Design review of the part built by this model. Coordinates are the model's own, in mm. A direction names the side the tool comes from. Give positions to 0.01 mm unless a question says otherwise; leave off trailing zeros. Write each loop counter-clockwise with the first axis right and the second up, starting at its lowest first coordinate (ties: lowest second). Pieces come first, ordered by that corner, then holes. Notation, with made-up numbers: (-23, 14.5) -> (8, 14.5) arc R30 cw to (8, 46.5) -> close; hole circle Ø2 at (87.5, -26). An arc over 180 degrees is marked (long way). Write each question's results on one line, items separated by ' | '. Start each with the question number.
(1) Mouldability with a two-part tool opening along Z and no side actions: class faces 1 (the face through (87, 1, 182)), 2 (the face through (80, 1, 195.7)), 3 (the face through (74, 0, 171)), 4 (the face through (80, 1, 197.7)) as released by +Z, released by -Z, zero draft, split by the parting line, or undercut.
(2) Take a section at A-A (z = 186). State the section outline as (x, y) points, plus the area to 3 significant figures.
(3) For faces 5 (the face through (71.4, 1, 190)), 6 (the face through (79.5, 2.2, 195.5)), list the 3-axis set-ups (+Z, -Z, +X, -X, +Y, -Y) from which the entire face can be reached by the end or side of a thin tool; tool diameter is ignored.
(4) Take a section at B-B (x = 81). State the section outline as (y, z) points.
(5) To check wall thickness, follow probe 1 along X at (y, z) = (0.35, 195); probe 2 along X at (y, z) = (0.3, 161); probe 3 along Z at (x, y) = (84, 0.9). State the ranges of each line that lie inside material, in increasing order.
(6) Take a section at D-D (z = 159). State the section outline as (x, y) points, plus the area to 3 significant figures.
(7) Take a section at C-C (y = 0.8). State the section outline as (x, z) points.
(8) Clearance check with flat-ended pins moving along their axes: pin 1 (1 mm diameter, centred on x = 83, z = 186, fed in from +Y); pin 2 (1.1 mm diameter, centred on x = 76.5, y = 1.5, fed in from -Z); pin 3 (1 mm diameter, centred on x = 85, y = 2, fed in from -Z); pin 4 (6 mm diameter, centred on x = 77, z = 185.5, fed in from -Y). State where each tip first meets the part, or that it passes through.
Autodesk Fusion 360 part; units mm, degrees
sketch "snippy-Edge_Cuts" plane through (0, 0, 0) normal (0, 1, 0) x (1, 0, 0)
  line L0 (73.4, -145) -> (85.6, -145)
  line L1 (85.6, -145) -> (85.6, -157)
  line L2 (85.6, -157) -> (73.4, -157)
  line L3 (73.4, -157) -> (73.4, -145)
  line L4 (73.4, -145) -> (73.4, -157)
  line L5 (73.4, -157) -> (85.6, -157)
  line L6 (85.6, -157) -> (85.6, -195.7)
  line L7 (85.6, -195.7) -> (73.4, -195.7)
  line L8 (73.4, -195.7) -> (73.4, -157)
  line L9 (87.6, -182) -> (87.6, -197.7)
  line L10 (87.6, -197.7) -> (71.4, -197.7)
  line L11 (71.4, -197.7) -> (71.4, -182)
  line L12 (73.4, -157) -> (85.6, -157)
  line L13 (84.5, -157) -> (74.5, -157)
  line L14 (74.5, -157) -> (74.5, -195.7)
  line L15 (74.5, -195.7) -> (84.5, -195.7)
  line L16 (84.5, -195.7) -> (84.5, -157)
  line L17 (85.6, -157) -> (85.6, -182)
  line L18 (85.6, -182) -> (87.6, -182)
  line L19 (87.6, -182) -> (71.4, -182)
  dimension "d4" = 12
  dimension "d8" = 12.2
  dimension "d9" = 12.2
  dimension "d23" = 10
  dimension "d25" = 1.1
  dimension "d26" = 1.1
extrude "Extrude6" add sketch "snippy-Edge_Cuts" along normal blind 0.4 contours L0 L1 L2 L3 L4 L5 L12 L13 | L2 L5 L8 L12 L14 L19 | L2 L5 L6 L12 L16 L17 L19 | L7 L8 L14 L19 | L6 L7 L8 L9 L10 L11 L15 L18 L19 | L6 L7 L16 L19 makes body 1
extrude "Extrude7" cut sketch "snippy-Edge_Cuts" along normal blind 2.6 contours L6 L7 L8 L9 L10 L11 L15 L18 L19 bodies 1
extrude "Extrude8" add sketch "snippy-Edge_Cuts" along normal blind 2.2 contours L6 L7 L8 L9 L10 L11 L15 L18 L19 bodies 1
extrude "Extrude9" add 1 faces at (77.4667, 2.2, 197.0333) along direction (0, 1, 0) blind 0.4 separate body on bodies 1 makes body 2
sketch "Sketch6" plane through (0, 2.6, 0) normal (0, 1, 0) x (-1, 0, 0)
  line L0 (-87.6, 197.7) -> (-87.6, 182)
  line L1 (-87.6, 182) -> (-85.6, 182)
  line L2 (-85.6, 182) -> (-85.6, 195.7)
  line L3 (-85.6, 195.7) -> (-73.4, 195.7)
  line L4 (-73.4, 195.7) -> (-73.4, 182)
  line L5 (-73.4, 182) -> (-71.4, 182)
  line L6 (-71.4, 182) -> (-71.4, 197.7)
  line L7 (-71.4, 197.7) -> (-87.6, 197.7)
  line L8 (-85.1, 182) -> (-85.1, 195.2)
  line L9 (-85.1, 195.2) -> (-73.9, 195.2)
  line L10 (-73.9, 195.2) -> (-73.9, 182)
  line L11 (-85.1, 182) -> (-85.6, 182)
  line L12 (-85.6, 182) -> (-85.6, 195.7)
  line L13 (-85.6, 195.7) -> (-73.4, 195.7)
  line L14 (-73.4, 195.7) -> (-73.4, 182)
  line L15 (-73.4, 182) -> (-73.9, 182)
  dimension "d40" = 0.5
extrude "Extrude10" add sketch "Sketch6" against normal blind 0.4 contours L2 L3 L4 L8 L9 L10 L11 L12 L13 L14 L15 bodies 1 2
fillet "Fillet2" radius 0.5 3 edges at (87.6, 2.6, 189.85) (79.5, 2.6, 197.7) (71.4, 2.6, 189.85) on bodies 1
sketch "Sketch3" plane through (0, 2.6, 0) normal (0, 1, 0) x (-1, 0, 0)
  line L0 (-85.6, 195.7) -> (-85.6, 157)
  line L1 (-73.4, 195.7) -> (-85.6, 195.7)
  line L2 (-73.4, 157) -> (-73.4, 195.7)
  line L3 (-85.6, 157) -> (-73.4, 157)
  line L4 (-85.1, 195.7) -> (-85.6, 195.7)
  line L5 (-73.9, 157) -> (-85.6, 157)
  line L6 (-85.6, 157) -> (-73.4, 157)
  line L7 (-73.4, 157) -> (-73.4, 195.7)
  line L8 (-73.4, 195.7) -> (-85.6, 195.7)
  line L9 (-73.9, 157) -> (-73.9, 195.2)
  line L10 (-73.9, 195.2) -> (-85.1, 195.2)
  line L11 (-85.1, 195.2) -> (-85.1, 157)
  dimension "d17" = 0.5
sketch "Sketch4" plane through (0, 0.4, 0) normal (0, 1, 0) x (-1, 0, 0)
  line L0 (-73.4, 145) -> (-73.4, 195.7)
  line L1 (-85.6, 195.7) -> (-85.6, 145)
  line L2 (-85.6, 145) -> (-73.4, 145)
  line L3 (-73.4, 195.7) -> (-85.6, 195.7)
Report:
1) face 1: released by -Z | face 2: undercut | face 3: zero draft | face 4: released by +Z
2) outline: (71.4, 0) -> (74.5, 0) -> (74.5, 0.4) -> (73.4, 0.4) -> (73.4, 2.2) -> (73.9, 2.2) -> (73.9, 2.6) -> (71.9, 2.6) arc R0.5 ccw to (71.4, 2.1) -> close; (84.5, 0) -> (87.6, 0) -> (87.6, 2.1) arc R0.5 ccw to (87.1, 2.6) -> (85.1, 2.6) -> (85.1, 2.2) -> (85.6, 2.2) -> (85.6, 0.4) -> (84.5, 0.4) -> close | area: 11.6 mm2
3) face 5: +Z, -Z, -X, +Y, -Y | face 6: -Z
4) outline: (0, 145) -> (0.4, 145) -> (0.4, 157) -> (0, 157) -> close; (0, 195.7) -> (2.2, 195.7) -> (2.2, 195.2) -> (2.6, 195.2) -> (2.6, 197.2) arc R0.5 ccw to (2.1, 197.7) -> (0, 197.7) -> close
5) probe 1: 71.4 to 74.5, 84.5 to 87.6 | probe 2: 73.4 to 74.5, 84.5 to 85.6 | probe 3: 195.7 to 197.7
6) outline: (73.4, 0) -> (74.5, 0) -> (74.5, 0.4) -> (73.4, 0.4) -> close; (84.5, 0) -> (85.6, 0) -> (85.6, 0.4) -> (84.5, 0.4) -> close | area: 0.880 mm2
7) outline: (71.4, 182) -> (73.4, 182) -> (73.4, 195.7) -> (85.6, 195.7) -> (85.6, 182) -> (87.6, 182) -> (87.6, 197.7) -> (71.4, 197.7) -> close
8) pin 1: through | pin 2: z = 195.7 | pin 3: z = 182 | pin 4: y = 0
